Check sheet for the modelled part. Datum: model origin and axes. Units: mm. A direction names the side the tool comes from. Round coordinates to 2 decimals unless told otherwise and drop trailing zeros. Order: outer loops, then holes, each group sorted by start corner. A loop starts at its lowest first (then second) coordinate and runs counter-clockwise, first axis right, second up. Notation, with made-up numbers: (53.25, 74) -> (112.25, 74) arc R16 ccw to (112.25, 101) -> close; hole circle Ø5 at (14, -8.75). An arc over 180 degrees is marked (long way). Answer in a Markdown table with one row per item. Add a question column.
1. Sectioned sample at A-A, the plane z = 0. Record the boundary of the cut face in (x, y), then the cut area to 3 significant figures.
2. Material ranges on L1, parallel to Z at x = 2.25, y = -1; L2, parallel to X at y = 0, z = -10.5; L3, parallel to X at y = -2.75, z = 2.5, recorded low to high. Write a range as from..to.
3. Access from +Z, -Z, +X, -X, +Y, -Y to the whole of each face (thin tool, end or side, straight path). Record for faces 1 (the flat face through (0.7, 1.5, 1.954)), 2 (the flat face through (0, 0, 3.954)).
4. Depth check by flat-ended pin: P1, Ø2, axis at y = 0.5, z = -7.5, coming from the -X side; P2, Ø2, axis at x = 1, z = -2, coming from the +Y side; P3, Ø1.5, axis at x = 1, z = -4.5, coming from the -Y side. Enter the tip coordinate at first touch or a pass-through.
Autodesk Inventor part; units mm, degrees
ref_plane "YZ Plane" through (0, 0, 0) normal (1, 0, 0) x (0, 1, 0)
ref_plane "XZ Plane" through (0, 0, 0) normal (0, 1, 0) x (-1, 0, 0)
ref_plane "XY Plane" through (0, 0, 0) normal (0, 0, 1) x (1, 0, 0)
sketch "Sketch1" plane through (0, 0, 0) normal (0, 1, 0) x (-1, 0, 0)
  line L0 (0, 3.9544) -> (10, 3.9544)
  line L1 (1.5, 1.9544) -> (1.5, -11.0456)
  line L2 (1.5, -11.0456) -> (0, -11.0456)
  line L3 (0, -11.0456) -> (0, 3.9544)
  line L4 (10, 3.9544) -> (10, 1.9544)
  line L5 (10, 1.9544) -> (1.5, 1.9544)
  point P0 (0, 0)
  dimension "d0" = 10
  dimension "d1" = 2
  dimension "d2" = 15
  dimension "d21" = 1.5
revolve "Revolution1" add sketch "Sketch1" angle 360 about axis through (0, 0, -11.0456) along (0, 0, 1)
thread "Thread2"
sketch "Sketch5" plane through (0, 0, 3.9544) normal (0, 0, 1) x (1, 0, 0)
  circle A0 centre (0, 0) radius 16.622
  line L0 (-2.9986, 1.7345) -> (0.0028, 3.4641)
  line L1 (0.0028, 3.4641) -> (3.0014, 1.7296)
  line L2 (3.0014, 1.7296) -> (2.9986, -1.7345)
  line L3 (2.9986, -1.7345) -> (-0.0028, -3.4641)
  line L4 (-0.0028, -3.4641) -> (-3.0014, -1.7296)
  line L5 (-3.0014, -1.7296) -> (-2.9986, 1.7345)
  dimension "d24" = 6
extrude "Extrusion1" cut sketch "Sketch5" against normal through all
fillet "Fillet1" radius 0.1 12 edges at (0.0028, 3.4641, 2.9544) (3.0014, 1.7296, 2.9544) (-2.9986, 1.7345, 2.9544) (2.9986, -1.7345, 2.9544) (-0.0028, -3.4641, 2.9544) (-3.0014, -1.7296, 2.9544) (1.5021, 2.5969, 3.9544) (-1.4979, 2.5993, 3.9544) (-3, 0.0024, 3.9544) (-1.5021, -2.5969, 3.9544) (1.4979, -2.5993, 3.9544) (3, -0.0024, 3.9544)
properties part number "Fi3es60mmcsavar" material "Steel, Alloy"
Answer key:
| question | item | result |
|---|---|---|
| 1 | outline | circle Ø3 at (0, 0) |
| 1 | area | 7.07 mm² |
| 2 | L1 | z = 1.95..3.95 |
| 2 | L2 | x = -1.5..1.5 |
| 2 | L3 | x = -1.24..1.24 |
| 3 | face 1 | -Z |
| 3 | face 2 | +Z, +X, -X, +Y, -Y |
| 4 | P1 | stops at x = -1.5 |
| 4 | P2 | stops at y = 1.5 |
| 4 | P3 | stops at y = -1.48 |
